from build123d import *

# Parameters (mm, degrees)
F0_R     = 9.5
F1_DEPTH = 14
F2_W     = 12
F2_H     = 49
F3_DEPTH = 6
F5_DEPTH = 106.001


with BuildPart() as f1:
    # F0 (on Front) → F1 (new body)
    with BuildSketch(Plane.XZ):
        Polygon((52.5, 25), (-53.5, 25), (-53.5, -24), (-2.5, -24), (52.5, 6), align=None)
        Circle(F0_R, mode=Mode.SUBTRACT)
    extrude(amount=F1_DEPTH)

    # F2 (on face) → F3 (join)
    with BuildSketch(Plane.XZ.offset(14)):
        with Locations((-47.5, 0.5)):
            Rectangle(F2_W, F2_H)
    extrude(amount=F3_DEPTH)

    # F4 (on face) → F5 (cut, through all)
    with BuildSketch(Plane(origin=(-53.5, 0, 0), x_dir=(0, -1, 0), z_dir=(-1, 0, 0))):
        Polygon((20, 25), (9, 25), (20, 14), align=None)
        Polygon((0, 25), (0, 20), (5, 25), align=None)
    extrude(amount=-F5_DEPTH, mode=Mode.SUBTRACT)


solid = f1.part
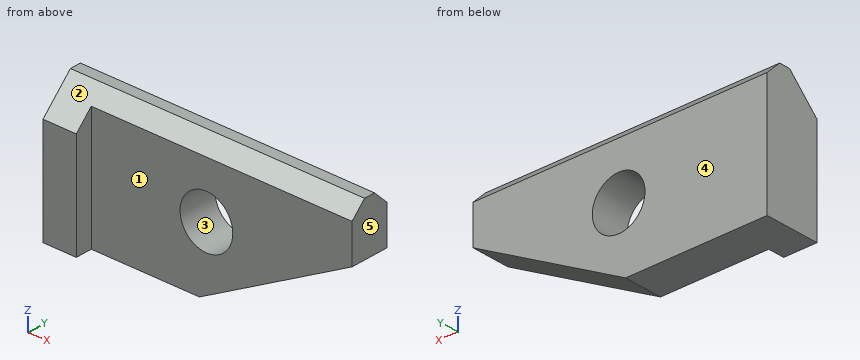
Read the model definition and answer for the solid it produces. Units are mm, in the model's axes. Face numbers are marked on the shaded views. A direction names the side the tool comes from. Round coordinates to 2 decimals unless told otherwise and drop trailing zeros. Write each loop counter-clockwise with the first axis right and the second up, starting at its lowest first coordinate (ties: lowest second). Pieces come first, ordered by that corner, then holes. Notation, with made-up numbers: M 77,57.25 L 133,57.25 A17 cw 133,77.25 Z; hole C -25,-36.5 d7. An arc over 180 degrees is marked long. Use a Markdown table: item, result.
1) The part is cut by section B-B (x = 0). Write down the section's boundary in (y, z), plus the area to 3 significant figures.
Answers follow:
| item | result |
|---|---|
| outline | M -14,-22.64 L 0,-22.64 L 0,-9.5 L -14,-9.5 Z; M -14,9.5 L 0,9.5 L 0,20 L -5,25 L -9,25 L -14,20 Z |
| area | 376 mm2 |
2) The part is cut by section A-A (z = 0). Write down the section's boundary in (x, y).
Answers follow:
| item | result |
|---|---|
| outline | M -53.5,-20 L -41.5,-20 L -41.5,-14 L -9.5,-14 L -9.5,0 L -53.5,0 Z; M 9.5,-14 L 41.5,-14 L 41.5,0 L 9.5,0 Z |
3) For a pull along X with two mould halves and no side action, classify the marked faces 3, 4 and 5 as pulls with the +X half, pulls with the -X half, needs draft (parallel to the pull), parting line crosses it, or undercut.
Answers follow:
| item | result |
|---|---|
| face 3 | undercut |
| face 4 | needs draft |
| face 5 | pulls with the +X half |
4) A tool of negligible diameter and unlimited length cuts with its end or side. For the marked faces 1 and 2, from which of +Z, -Z, +X, -X, +Y, -Y can it reach the whole face along a straight path? Write none if from no direction.
Answers follow:
| item | result |
|---|---|
| face 1 | +Z, -Z, +X, -Y |
| face 2 | +Z, +X, -X, -Y |
5) Flat-ended cylindrical pins translate along their axes: pin 1 (1.5 mm diameter, centred on x = -4.5, y = -2.5, fed in from +Z); pin 2 (3 mm diameter, centred on x = 13, y = -12, fed in from +Z); pin 3 (1 mm diameter, centred on x = -20.5, z = 20, fed in from -Y). Find the tip coordinate at first contact, or state that the pin passes through.
Answers follow:
| item | result |
|---|---|
| pin 1 | stops at z = 23.25 |
| pin 2 | stops at z = 23.5 |
| pin 3 | stops at y = -14 |
6) The part is cut by section C-C (y = -12.5). Write down the section's boundary in (x, z), plus the area to 3 significant figures.
Answers follow:
| item | result |
|---|---|
| outline | M -53.5,-24 L -2.5,-24 L 52.5,6 L 52.5,21.5 L -53.5,21.5 Z; hole C 0,0 d19 |
| area | 3,710 mm2 |
7) The part is cut by section D-D (z = -15). Write down the section's boundary in (x, y).
Answers follow:
| item | result |
|---|---|
| outline | M -53.5,-20 L -41.5,-20 L -41.5,-14 L 14,-14 L 14,0 L -53.5,0 Z |
8) Straight lines are drawn through the part: line 1 along Y through (x, z) = (-8.5, 5); line 2 along Z through (x, y) = (0, -4.25); line 3 along Z through (x, y) = (0, -10). For each, find the intervals that lie inside material, in ascending order. Write a range as [from, to].
Answers follow:
| item | result |
|---|---|
| line 1 | y = [-14, 0] |
| line 2 | z = [-22.64, -9.5], [9.5, 24.25] |
| line 3 | z = [-22.64, -9.5], [9.5, 24] |
